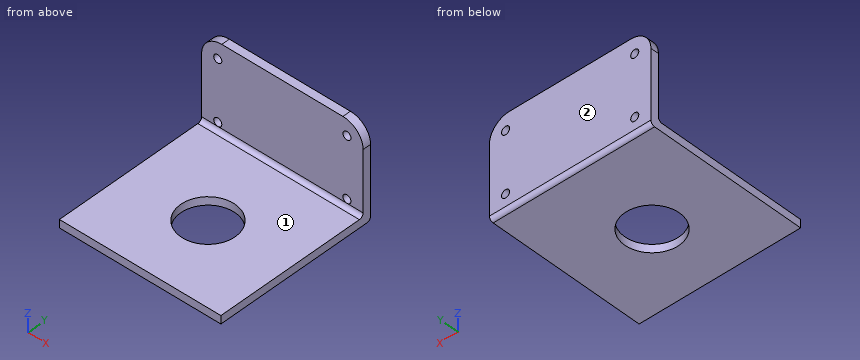
from build123d import *

# Parameters (mm, degrees)
SKETCH1_W           = 40
SKETCH1_H           = 40
SKETCH1_R           = 6.75
BOSS_EXTRUDE2_DEPTH = 2
SKETCH2_W           = 40
SKETCH2_H           = 2
BOSS_EXTRUDE3_DEPTH = 23
SKETCH3_R           = 1
CUT_EXTRUDE1_DEPTH  = 2
FILLET1_R           = 1
FILLET2_R           = 1
FILLET3_R           = 5


with BuildPart() as part:
    # Sketch1 → Boss-Extrude2 (new body)
    with BuildSketch(Plane.XY):
        Rectangle(SKETCH1_W, SKETCH1_H)
        with Locations((0, -1.878854291)):
            Circle(SKETCH1_R, mode=Mode.SUBTRACT)
    extrude(amount=BOSS_EXTRUDE2_DEPTH)

    # Sketch2 → Boss-Extrude3 (add)
    with BuildSketch(Plane.XY):
        with Locations((0, 19)):
            Rectangle(SKETCH2_W, SKETCH2_H)
    extrude(amount=BOSS_EXTRUDE3_DEPTH)

    # Sketch3 → Cut-Extrude1 (cut)
    with BuildSketch(Plane(origin=(0, 20, 0), x_dir=(1, 0, 0), z_dir=(0, 1, 0))):
        with Locations(Location((-16, -4, 0), (0, 0, 270))):
            Circle(SKETCH3_R)
        with Locations(Location((16, -4, 0), (0, 0, 270))):
            Circle(SKETCH3_R)
        with Locations(Location((16, -19, 0), (0, 0, 270))):
            Circle(SKETCH3_R)
        with Locations(Location((-16, -19, 0), (0, 0, 270))):
            Circle(SKETCH3_R)
    extrude(amount=-CUT_EXTRUDE1_DEPTH, mode=Mode.SUBTRACT)

    # Fillet1
    fillet1_edges = [part.edges().sort_by_distance(p)[0] for p in [
        (0, 20, 0),
    ]]
    fillet(fillet1_edges, radius=FILLET1_R)

    # Fillet2
    fillet2_edges = [part.edges().sort_by_distance(p)[0] for p in [
        (0, 18, 2),
    ]]
    fillet(fillet2_edges, radius=FILLET2_R - 0.0001)  # a hair under: the kernel refuses the full size

    # Fillet3
    fillet3_edges = [part.edges().sort_by_distance(p)[0] for p in [
        (-20, 19, 23),
        (20, 19, 23),
    ]]
    fillet(fillet3_edges, radius=FILLET3_R)


solid = part.part
Check sheet for the modelled part. Datum: model origin and axes. Units: mm. Face numbers are marked on the shaded views. A direction names the side the tool comes from. Give positions to 0.01 mm unless a question says otherwise; leave off trailing zeros. Loops run counter-clockwise (first coordinate to the right, second up) from the corner with the lowest first, then second, coordinate; pieces in that order, holes last. Notation, with made-up numbers: M -10,42 L -5,42 A32 ccw -5,76 Z; hole C 85,8.25 d6. An arc over 180 degrees is marked long. Use a Markdown table: item, result. Add a question column.
Q1. Go/stop test with flat-tipped pins: pin 1 (3 mm diameter, centred on x = 16, z = 19, fed in from -Y); pin 2 (1.2 mm diameter, centred on x = 16, z = 4, fed in from +Y); pin 3 (12 mm diameter, centred on x = -15.5, y = -16, fed in from +Z); pin 4 (2.5 mm diameter, centred on x = -16, z = 4, fed in from +Y). Record where each tip stops, or that it passes through.
Q2. Sectioned sample at B-B, the plane y = 3.5. Record the cut outline in (x, z), then the cut area to 3 significant figures.
Q3. Sectioned sample at D-D, the plane z = 19. Record the cut outline in (x, y).
Q4. Scan lines: line 1 along X through (y, z) = (19.25, 4); line 2 along X through (y, z) = (19.5, 19); line 3 along Z through (x, y) = (6, 4). Record each from-to range of solid material in increasing order. Write a range as [from, to].
Q5. Sectioned sample at A-A, the plane x = 0. Record the cut outline in (y, z).
Q6. Sectioned sample at C-C, the plane x = 9. Record the cut outline in (y, z).
Q7. Tool access check on the marked faces 1 and 2. Record the directions out of +Z, -Z, +X, -X, +Y, -Y that give a thin tool (end or side, any length) a straight path to the whole face; none if there is none.
Verdict:
| question | item | result |
|---|---|---|
| 1 | pin 1 | y = 18 |
| 1 | pin 2 | through |
| 1 | pin 3 | z = 2 |
| 1 | pin 4 | y = 20 |
| 2 | outline | M -20,0 L -4.08,0 L -4.08,2 L -20,2 Z; M 4.08,0 L 20,0 L 20,2 L 4.08,2 Z |
| 2 | area | 63.7 mm^2 |
| 3 | outline | M -19.9,18 L -17,18 L -17,20 L -19.9,20 Z; M -15,18 L 15,18 L 15,20 L -15,20 Z; M 17,18 L 19.9,18 L 19.9,20 L 17,20 Z |
| 4 | line 1 | [-20, -17], [-15, 15], [17, 20] |
| 4 | line 2 | [-19.9, -17], [-15, 15], [17, 19.9] |
| 4 | line 3 | [0, 2] |
| 5 | outline | M -20,0 L -8.63,0 L -8.63,2 L -20,2 Z; M 4.87,0 L 19,0 A1 ccw 20,1 L 20,23 L 18,23 L 18,3 A1 cw 17,2 L 4.87,2 Z |
| 6 | outline | M -20,0 L 19,0 A1 ccw 20,1 L 20,23 L 18,23 L 18,3 A1 cw 17,2 L -20,2 Z |
| 7 | face 1 | +Z, +X, -X, -Y |
| 7 | face 2 | +Z, -Z, +X, -X, +Y |
